```python
from build123d import *

# Parameters (mm, degrees)
SKETCH1_W                    = 10
SKETCH1_H                    = 70
BOSS_EXTRUDE1_DEPTH          = 9.5
SKETCH2_W                    = 54.25
SKETCH2_H                    = 9.5
CUT_EXTRUDE1_DEPTH           = 38.619808612
SKETCH3_R                    = 1.475
CUT_EXTRUDE2_DEPTH           = 37.609425016
SKETCH4_W                    = 10
SKETCH4_H                    = 9.875
SKETCH4_R                    = 1.475
BOSS_EXTRUDE2_DEPTH          = 2
BODY_DELETE_KEEP_2_OUTLINE_W = 10
BODY_DELETE_KEEP_2_OUTLINE_H = 9.875
BODY_DELETE_KEEP_2_OUTLINE_R = 1.475
BODY_DELETE_KEEP_2_DEPTH     = 11.5
BODY_MOVE_COPY1_ANGLE        = 90


with BuildPart() as part:
    # Sketch1 → Boss-Extrude1 (new body)
    with BuildSketch(Plane(origin=(0, 0, 0), x_dir=(1, 0, 0), z_dir=(0, 1, 0))):
        Rectangle(SKETCH1_W, SKETCH1_H)
    extrude(amount=BOSS_EXTRUDE1_DEPTH)

    # Sketch2 → Cut-Extrude1 (cut, through all)
    with BuildSketch(Plane(origin=(5, 0, 0), x_dir=(0, 0, -1), z_dir=(1, 0, 0))):
        with Locations((0, 4.75)):
            Rectangle(SKETCH2_W, SKETCH2_H)
    extrude(amount=-CUT_EXTRUDE1_DEPTH, mode=Mode.SUBTRACT)


with BuildPart() as cut_extrude1_piece_1:
    # of the separate pieces the step leaves, piece 1, a body of its own (cut_extrude1_pieces)
    add(part.part.solids().sort_by_distance((-5, 0, 35))[0])


with BuildPart() as cut_extrude1_piece_2:
    # of the separate pieces the step leaves, piece 2, a body of its own (cut_extrude1_pieces)
    add(part.part.solids().sort_by_distance((-5, 0, -35))[0])


with BuildPart() as cut_extrude2_tool:
    # Sketch3 → Cut-Extrude2 (new, through all)
    with BuildSketch(Plane.XZ):
        with Locations(Location((0, 30, 0), (0, 0, 270))):
            Circle(SKETCH3_R)
        with Locations(Location((0, -30, 0), (0, 0, 270))):
            Circle(SKETCH3_R)
    extrude(amount=-CUT_EXTRUDE2_DEPTH)


with BuildPart() as cut_extrude1_piece_1_1:
    add(cut_extrude1_piece_1.part)

    # Cut-Extrude2: cut by cut_extrude2_tool
    add(cut_extrude2_tool.part, mode=Mode.SUBTRACT)



with BuildPart() as cut_extrude1_piece_2_1:
    add(cut_extrude1_piece_2.part)

    # Cut-Extrude2: cut by cut_extrude2_tool
    add(cut_extrude2_tool.part, mode=Mode.SUBTRACT)


with BuildPart() as cut_extrude1_piece_1_2:
    add(cut_extrude1_piece_1_1.part)

    add(cut_extrude1_piece_2_1.part)  # Boss-Extrude2 merges Cut-Extrude1 piece 2
    # Sketch4 → Boss-Extrude2 (add)
    # profile 1 of 2: a face of its own
    with BuildSketch(Plane(origin=(0, 9.5, 0), x_dir=(1, 0, 0), z_dir=(0, 1, 0))):
        with Locations((0, -30.0625)):
            Rectangle(SKETCH4_W, SKETCH4_H)
        with Locations(Location((0, -30, 0), (0, 0, 90))):
            Circle(SKETCH4_R, mode=Mode.SUBTRACT)
    # profile 2 of 2: a face of its own
    with BuildSketch(Plane(origin=(0, 9.5, 0), x_dir=(1, 0, 0), z_dir=(0, 1, 0))):
        with Locations((0, 30.0625)):
            Rectangle(SKETCH4_W, SKETCH4_H)
        with Locations(Location((0, 30, 0), (0, 0, 90))):
            Circle(SKETCH4_R, mode=Mode.SUBTRACT)
    extrude(amount=BOSS_EXTRUDE2_DEPTH)

    # Body-Delete/Keep 2: read off the stored shape, not the designer's step
    # Body-Delete/Keep 2 outline → Body-Delete/Keep 2 (cut)
    with BuildSketch(Plane(origin=(0, 0, 0), x_dir=(1, 0, 0), z_dir=(0, 1, 0))):
        with Locations((0, 30.0625)):
            Rectangle(BODY_DELETE_KEEP_2_OUTLINE_W, BODY_DELETE_KEEP_2_OUTLINE_H)
        with Locations((0, 30)):
            Circle(BODY_DELETE_KEEP_2_OUTLINE_R, mode=Mode.SUBTRACT)
    extrude(amount=BODY_DELETE_KEEP_2_DEPTH, mode=Mode.SUBTRACT)


with BuildPart() as cut_extrude1_piece_1_3:
    # Body-Move/Copy1: read off the stored shape, not the designer's step
    # Body-Move/Copy1: moved
    add(cut_extrude1_piece_1_2.part.moved(Location((0, -11.5, 11.5))).rotate(Axis((0, 0, 0), (-1, 0, 0)), BODY_MOVE_COPY1_ANGLE))


solid = cut_extrude1_piece_1_3.part
```
Could you check a few things on this model? Use its own coordinates, in mm. Give positions to 0.01 mm unless a question says otherwise; leave off trailing zeros. Write each loop counter-clockwise with the first axis right and the second up, starting at its lowest first coordinate (ties: lowest second). Pieces come first, ordered by that corner, then holes. Notation, with made-up numbers: (10, 28.25) - (61, 28.25) arc R13 ccw to (61, 47.25) - close; hole circle Ø8 at (83.5, 74). An arc over 180 degrees is marked (long way). One line per item, written item: value. Start each with the question number.
Item 1: Imagine slicing it at B-B, the plane y = 41.5. List the corners of the cut face in (x, z) for me (3 decimals).
Item 2: Imagine slicing it at C-C, the plane z = 1.25. List the corners of the cut face in (x, y) for me (3 decimals).
Item 3: Imagine slicing it at A-A, the plane x = 0. List the corners of the cut face in (y, z) for me (3 decimals), and give its area (3 significant figures).
Item 4: Please list where these lines run through material, in increasing order: line 1 (X direction, y = 41.5, z = 7.25) (3 decimals); line 2 (Y direction, x = 0, z = 5.75) (3 decimals); line 3 (Z direction, x = 0.25, y = 37.5). Write a range as from..to.
Item 5: Imagine slicing it at D-D, the plane x = 2.5. List the corners of the cut face in (y, z) for me (3 decimals).
Item 6: If we mould it in two halves opening along Y, with no side actions, what happens to faces 1 (the face through (0, 38.625, 7)), 2 (the face through (0.565, 40.137, 5.831)), 3 (the face through (0, 38, 2))? For each: +Y half, -Y half, draft (parallel to the pull), parting line (faces both ways), or undercut.
Item 7: I'm going to push flat-ended pins straight in: pin 1 (1 mm diameter, centred on x = -0.5, z = 6.5, fed in from -Y) (3 decimals); pin 2 (1 mm diameter, centred on x = -0.5, y = 38, fed in from +Z). Where does each tip first touch, or does it pass through?
Geometry says:
1. outline: (-5, 0) - (-1.475, 0) - (-1.475, 11.5) - (-5, 11.5) - close; (1.475, 0) - (5, 0) - (5, 11.5) - (1.475, 11.5) - close
2. outline: (-5, 36.625) - (5, 36.625) - (5, 46.5) - (-5, 46.5) - close; hole circle Ø2.95 at (0, 41.5)
3. outline: (36.625, 0) - (40.025, 0) - (40.025, 11.5) - (38.625, 11.5) - (38.625, 2) - (36.625, 2) - close; (42.975, 0) - (46.5, 0) - (46.5, 11.5) - (42.975, 11.5) - close
3. area: 60.6 mm^2
4. line 1: -5..-1.475, 1.475..5
4. line 2: 38.625..40.025, 42.975..46.5
4. line 3: 0..2
5. outline: (36.625, 0) - (46.5, 0) - (46.5, 11.5) - (38.625, 11.5) - (38.625, 2) - (36.625, 2) - close
6. face 1: -Y half
6. face 2: undercut
6. face 3: draft
7. pin 1: y = 38.625
7. pin 2: z = 2
